For this review, use the dimensioned drawing (mm, ordinates from the lowest corner) and the shaded views. Round coordinates to 2 decimals unless told otherwise and drop trailing zeros. Loops run counter-clockwise (first coordinate to the right, second up) from the corner with the lowest first, then second, coordinate; pieces in that order, holes last. Notation, with made-up numbers: (40, 8) - (58, 8) arc R19 cw to (58, 37) - close; hole circle Ø1 at (66.5, 37). An arc over 180 degrees is marked (long way). Return JSON: item names as keys, results as strings. Group by question number.
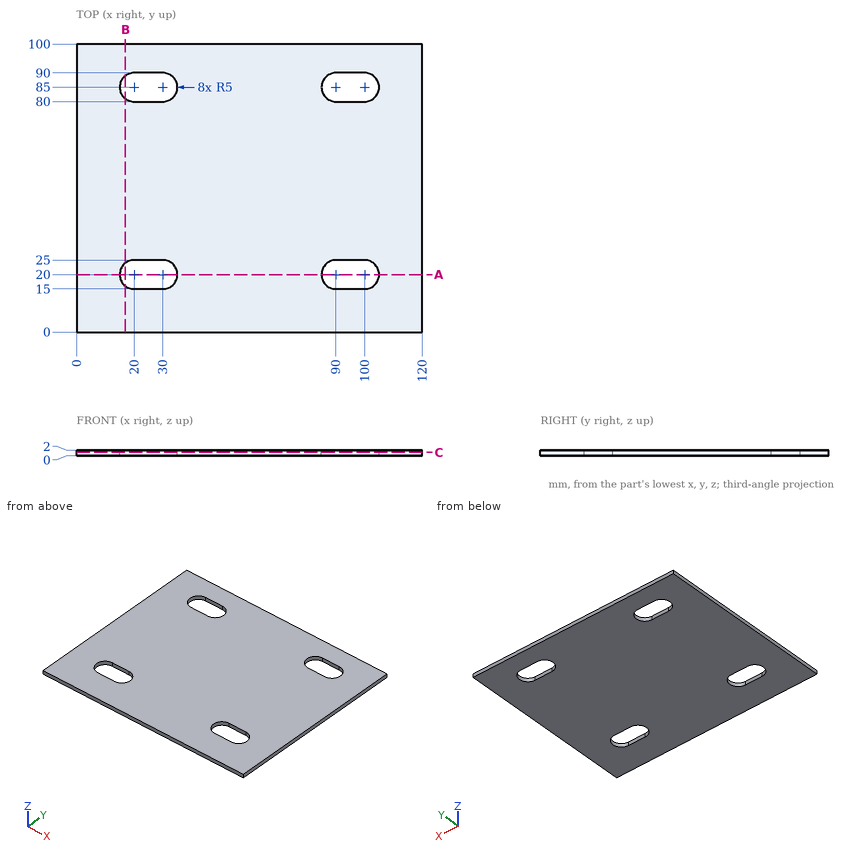
Q1. For line 1 (Y direction, x = 21, z = 0.8); line 2 (X direction, y = 24, z = 0.8); line 3 (X direction, y = 83, z = 0.95), list the stretches that pass through material, from the lowest coordinate up.
Q2. Add section C-C, the plane z = 1.2. State the section outline as (x, y) points, plus the area to 3 significant figures.
Q3. Add section B-B, the plane x = 17. State the section outline as (y, z) points.
Q4. Add section A-A, the plane y = 20. State the section outline as (x, z) points, plus the area to 3 significant figures.
Evaluation:
{
 "1": {"line 1": "0 to 15, 25 to 80, 90 to 100", "line 2": "0 to 17, 33 to 87, 103 to 120", "line 3": "0 to 15.42, 34.58 to 85.42, 104.58 to 120"},
 "2": {"outline": "(0, 0) - (120, 0) - (120, 100) - (0, 100) - close; hole (20, 15) - (30, 15) arc R5 ccw to (30, 25) - (20, 25) arc R5 ccw to start; hole (20, 80) - (30, 80) arc R5 ccw to (30, 90) - (20, 90) arc R5 ccw to start; hole (90, 15) - (100, 15) arc R5 ccw to (100, 25) - (90, 25) arc R5 ccw to start; hole (90, 80) - (100, 80) arc R5 ccw to (100, 90) - (90, 90) arc R5 ccw to start", "area": "11,300 mm²"},
 "3": {"outline": "(0, 0) - (16, 0) - (16, 2) - (0, 2) - close; (24, 0) - (81, 0) - (81, 2) - (24, 2) - close; (89, 0) - (100, 0) - (100, 2) - (89, 2) - close"},
 "4": {"outline": "(0, 0) - (15, 0) - (15, 2) - (0, 2) - close; (35, 0) - (85, 0) - (85, 2) - (35, 2) - close; (105, 0) - (120, 0) - (120, 2) - (105, 2) - close", "area": "160 mm²"}
}
